```python
from build123d import *

# Parameters (mm, degrees)
EXTRUDE_1_DEPTH     = 3
SKETCH_2_R          = 1.6
CUT_EXTRUDE_1_DEPTH = 10


with BuildPart() as part:
    # 草图1 → 凸台-拉伸1 (new body)
    with BuildSketch(Plane.XY):
        Polygon((60, 0), (0, 0), (0, 20), (20, 20), (0.947441117, 31), (10.947441117, 48.320508076), (60, 20), align=None)
    extrude(amount=EXTRUDE_1_DEPTH)

    # 草图2 → 切除-拉伸1 (cut)
    with BuildSketch(Plane.XY.offset(3)):
        with Locations((13.643593539, 40.990381057)):
            Circle(SKETCH_2_R)
        with Locations((8.643593539, 32.330127019)):
            Circle(SKETCH_2_R)
        with Locations((24.035898385, 34.990381057)):
            Circle(SKETCH_2_R)
        with Locations((19.035898385, 26.330127019)):
            Circle(SKETCH_2_R)
        with Locations((6, 16)):
            Circle(SKETCH_2_R)
        with Locations((6, 4)):
            Circle(SKETCH_2_R)
        with Locations((54, 16)):
            Circle(SKETCH_2_R)
        with Locations((54, 4)):
            Circle(SKETCH_2_R)
        with Locations((16, 16)):
            Circle(SKETCH_2_R)
        with Locations((16, 4)):
            Circle(SKETCH_2_R)
        with Locations((44, 16)):
            Circle(SKETCH_2_R)
        with Locations((44, 4)):
            Circle(SKETCH_2_R)
        with BuildLine():
            Line((21, 14), (39, 14))
            ThreePointArc((39, 14), (43, 10), (39, 6))
            Line((39, 6), (21, 6))
            ThreePointArc((21, 6), (17, 10), (21, 14))
        make_face()
    extrude(amount=-CUT_EXTRUDE_1_DEPTH, mode=Mode.SUBTRACT)


solid = part.part
```
CAD build for the part. Positions are in the model's coordinates, mm. A direction names the side the tool comes from. Round coordinates to 2 decimals unless told otherwise and drop trailing zeros. Loops run counter-clockwise (first coordinate to the right, second up) from the corner with the lowest first, then second, coordinate; pieces in that order, holes last. Notation, with made-up numbers: (86, 10.5) - (108, 10.5) arc R29 ccw to (108, 41.5) - close; hole circle Ø1 at (-25.75, -28). An arc over 180 degrees is marked (long way). Return JSON: item names as keys, results as strings. Group by question number.
Q1. Band-saw the part on D-D on x = 54. Give the cut face in (y, z).
Q2. Drill centre lines: line 1 along Y through (x, z) = (16, 0.75); line 2 along Y through (x, z) = (53.5, 1.4); line 3 along Y through (x, z) = (44, 0.7). Where is each one in solid material? Low to high. Write a range as [from, to].
Q3. Band-saw the part on C-C on x = 27.5. Give the cut face in (y, z), plus the area to 3 significant figures.
Q4. Two-plate mould, pull along Y, no slides. Class faces 4 (the face through (30, 19, 3)), 5 (the face through (55.526, 4.481, 1.521)), 6 (the face through (35.13, 34.36, 1.48)): +Y half, -Y half, draft (parallel to the pull), parting line (faces both ways), or undercut.
Q5. Flat gauge pins, fed straight in: pin 1 Ø5 at (x, y) = (6, 16) entering from -Z; pin 2 Ø1.5 at (x, z) = (29, 2) entering from +Y; pin 3 Ø1.5 at (y, z) = (33.5, 1.5) entering from -X; pin 4 Ø1 at (y, z) = (31.5, 2) entering from +X. Where does each tip first touch, or does it go through?
Q6. Tool access for faces 1 (the face through (30, 0, 1)), 2 (the face through (30, 6, 2)), 3 (the face through (10.61, 25.42, 1.48)): list every direction of +Z, -Z, +X, -X, +Y, -Y with a clear straight run to the whole face (end or side of a thin tool).
Q7. Band-saw the part on B-B on y = 10. Give the cut face in (x, z), plus the area to 3 significant figures.
Q8. Band-saw the part on A-A on y = 4. Give the cut face in (x, z).
Solutions:
{
 "1": {"outline": "(0, 0) - (2.4, 0) - (2.4, 3) - (0, 3) - close; (5.6, 0) - (14.4, 0) - (14.4, 3) - (5.6, 3) - close; (17.6, 0) - (23.46, 0) - (23.46, 3) - (17.6, 3) - close"},
 "2": {"line 1": "y = [0, 2.4], [5.6, 14.4], [17.6, 20], [22.31, 45.4]", "line 2": "y = [0, 2.48], [5.52, 14.48], [17.52, 23.75]", "line 3": "y = [0, 2.4], [5.6, 14.4], [17.6, 29.24]"},
 "3": {"outline": "(0, 0) - (6, 0) - (6, 3) - (0, 3) - close; (14, 0) - (38.76, 0) - (38.76, 3) - (14, 3) - close", "area": "92.3 mm^2"},
 "4": {"face 4": "draft", "face 5": "undercut", "face 6": "+Y half"},
 "5": {"pin 1": "stops at z = 0", "pin 2": "stops at y = 38.33", "pin 3": "stops at x = 1.96", "pin 4": "stops at x = 40.95"},
 "6": {"face 1": "+Z, -Z, +X, -X, -Y", "face 2": "+Z, -Z", "face 3": "+Z, -Z, -X"},
 "7": {"outline": "(0, 0) - (17, 0) - (17, 3) - (0, 3) - close; (43, 0) - (60, 0) - (60, 3) - (43, 3) - close", "area": "102 mm^2"},
 "8": {"outline": "(0, 0) - (4.4, 0) - (4.4, 3) - (0, 3) - close; (7.6, 0) - (14.4, 0) - (14.4, 3) - (7.6, 3) - close; (17.6, 0) - (42.4, 0) - (42.4, 3) - (17.6, 3) - close; (45.6, 0) - (52.4, 0) - (52.4, 3) - (45.6, 3) - close; (55.6, 0) - (60, 0) - (60, 3) - (55.6, 3) - close"}
}
